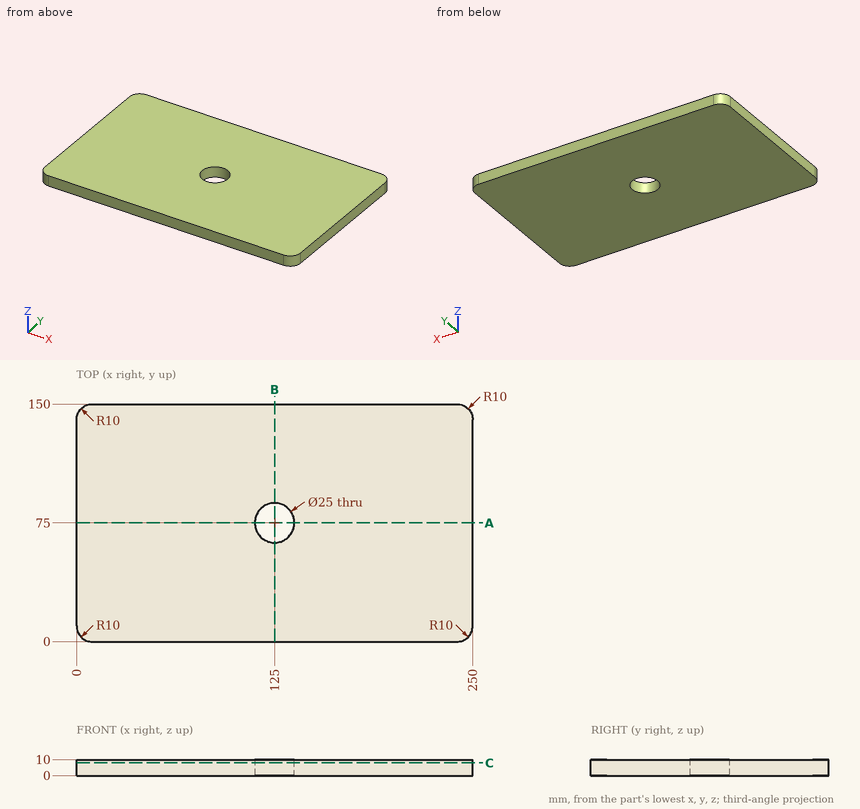
Geometry: see drawing. Coordinates: mm, zero at the bounding-box minimum. Coordinates: 2 decimals unless noted, no trailing zeros. Loops run counter-clockwise (first coordinate to the right, second up) from the corner with the lowest first, then second, coordinate; pieces in that order, holes last.
Q1. Material intervals for line 1 (Y direction, x = 125, z = 3.25); line 2 (Y direction, x = 136, z = 9.5), sorted ascending.
Q2. Cut plane A-A (y = 75). Output: boundary loops of the cut face in (x, z), then the cut area to 3 significant figures.
Q3. Cut plane B-B (x = 125). Output: boundary loops of the cut face in (y, z), then the cut area to 3 significant figures.
Q4. Cut plane C-C (z = 8). Output: boundary loops of the cut face in (x, y), then the cut area to 3 significant figures.
Working result:
1. line 1: y = 0 to 62.5, 87.5 to 150
1. line 2: y = 0 to 69.06, 80.94 to 150
2. outline: (0, 0) - (112.5, 0) - (112.5, 10) - (0, 10) - close; (137.5, 0) - (250, 0) - (250, 10) - (137.5, 10) - close
2. area: 2,250 mm2
3. outline: (0, 0) - (62.5, 0) - (62.5, 10) - (0, 10) - close; (87.5, 0) - (150, 0) - (150, 10) - (87.5, 10) - close
3. area: 1,250 mm2
4. outline: (0, 10) arc R10 ccw to (10, 0) - (240, 0) arc R10 ccw to (250, 10) - (250, 140) arc R10 ccw to (240, 150) - (10, 150) arc R10 ccw to (0, 140) - close; hole circle Ø25 at (125, 75)
4. area: 36,900 mm2
